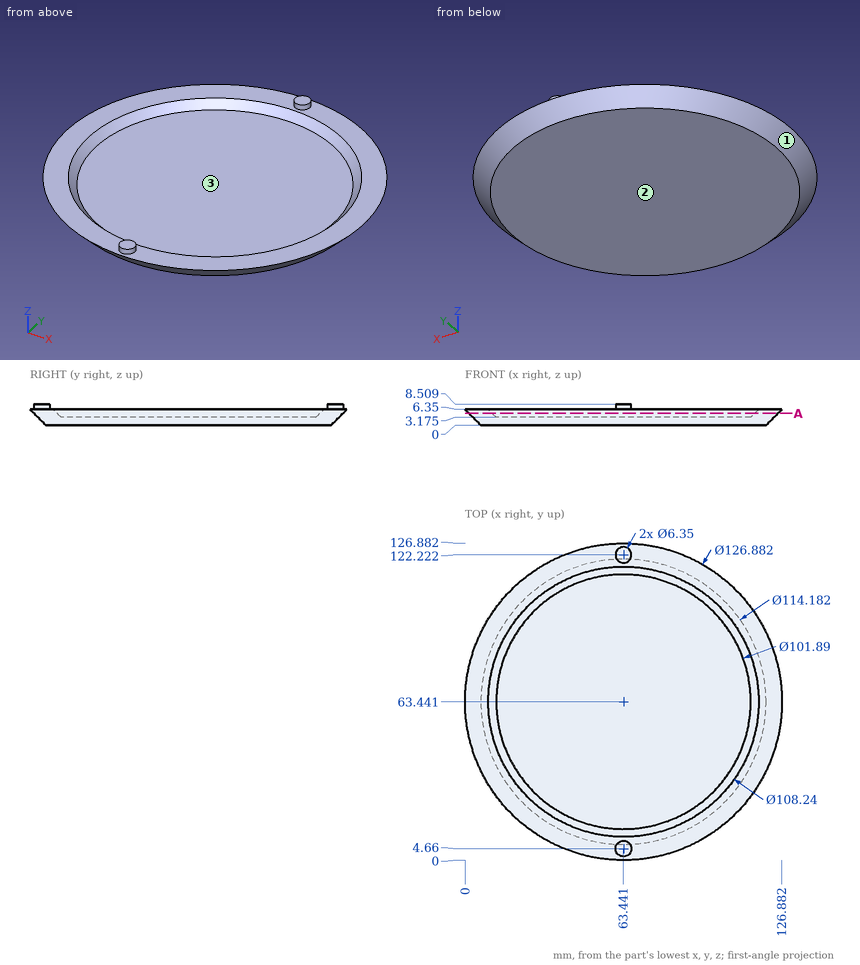
Drawing for the job (mm, zero at the part's lowest x, y, z). Round coordinates to 2 decimals unless told otherwise and drop trailing zeros. Order: outer loops, then holes, each group sorted by start corner. A loop starts at its lowest first (then second) coordinate and runs counter-clockwise, first axis right, second up.
Item 1: Probe line 1 along Z through (x, y) = (26.5, 91) (1 decimal); line 2 along X through (y, z) = (50.5, 4) (1 decimal); line 3 along X through (y, z) = (33, 6) (1 decimal). List the from-to ranges inside material, lowest first.
Item 2: Pin check, flat tips, straight feed: pin 1 (5 mm diameter, centred on y = 88, z = 6, fed in from +X) (1 decimal); pin 2 (3 mm diameter, centred on y = 76.5, z = 1.5, fed in from +X); pin 3 (1.5 mm diameter, centred on y = 36, z = 3, fed in from +X). Stop position of each tip, or through.
Item 3: Mould opens along Y. For the marked faces 1, 2 and 3 say: pulls with the +Y half, pulls with the -Y half, needs draft (parallel to the pull), parting line crosses it, or undercut.
Item 4: Saw through at A-A on z = 4.75. Write the cut outline in (x, y), then the cut area to 3 significant figures.
Reported:
1. line 1: z = 0 to 3.2
1. line 2: x = 3.7 to 13.3, 113.6 to 123.1
1. line 3: x = 8.2 to 19.1, 107.8 to 118.7
2. pin 1: stops at x = 122.9
2. pin 2: stops at x = 122.13
2. pin 3: stops at x = 117.82
3. face 1: parting line crosses it
3. face 2: needs draft
3. face 3: undercut
4. outline: circle Ø123.68 at (63.44, 63.44); hole circle Ø105.04 at (63.44, 63.44)
4. area: 3,350 mm2
